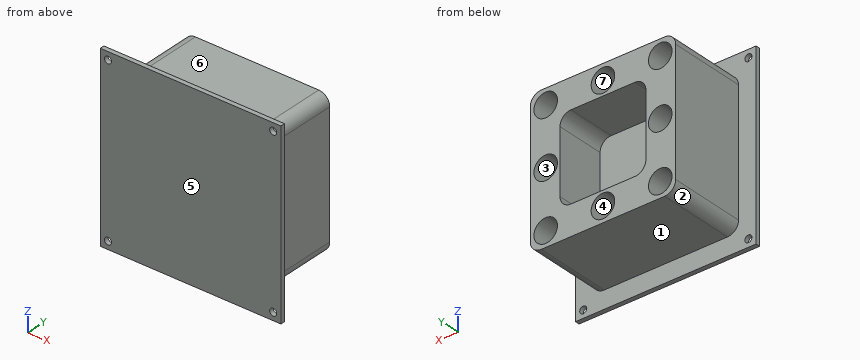
Autodesk Inventor part; units mm, degrees
ref_plane "YZ Plane" through (0, 0, 0) normal (1, 0, 0) x (0, 1, 0)
ref_plane "XZ Plane" through (0, 0, 0) normal (0, 1, 0) x (-1, 0, 0)
ref_plane "XY Plane" through (0, 0, 0) normal (0, 0, 1) x (1, 0, 0)
sketch "Sketch1" plane through (0, 0, 0) normal (0, 1, 0) x (-1, 0, 0)
  line L0 (28, 33) -> (-28, 33)
  line L1 (-33, 28) -> (-33, -28)
  line L2 (-28, -33) -> (28, -33)
  line L3 (33, -28) -> (33, 28)
  line L4 (33, 33) -> (-33, -33) construction
  line L5 (-33, 33) -> (33, -33) construction
  arc A0 (28, -33) -> (33, -28) centre (28, -28) ccw
  arc A1 (33, 28) -> (28, 33) centre (28, 28) ccw
  arc A2 (-28, 33) -> (-33, 28) centre (-28, 28) ccw
  arc A3 (-33, -28) -> (-28, -33) centre (-28, -28) ccw
  point P0 (0, 0)
  dimension "d0" = 66
  dimension "d1" = 66
  dimension "d4" = 5
extrude "Extrusion1" add sketch "Sketch1" along normal blind 35
sketch "Sketch2" plane through (0, 35, 0) normal (0, 1, 0) x (1, 0, 0)
  line L0 (0, 0) -> (-10, 0)
  line L1 (0, 0) -> (0, -10)
  circle A0 centre (26, 26) radius 5.35
  circle A1 centre (0, 26) radius 5.35
  circle A2 centre (-26, 26) radius 5.35
  circle A3 centre (26, 0) radius 5.35
  circle A4 centre (0, 0) radius 5.35
  circle A5 centre (-26, 0) radius 5.35
  circle A6 centre (26, -26) radius 5.35
  circle A7 centre (0, -26) radius 5.35
  circle A8 centre (-26, -26) radius 5.35
  dimension "d8" = 10
  dimension "d9" = 10
  dimension "d10" = 10.7
  dimension "d11" = 26
  dimension "d12" = 26
  dimension "d15" = 26
  dimension "d18" = 26
extrude "Extrusion2" cut sketch "Sketch2" against normal blind 35 contours A0 | A1 | A2 | A3 | A5 | A6 | A7 | A8
sketch "Sketch3" plane through (0, 35, 0) normal (0, 1, 0) x (1, 0, 0)
  line L0 (-14.5, -19.5) -> (14.5, -19.5)
  line L1 (19.5, -14.5) -> (19.5, 14.5)
  line L2 (14.5, 19.5) -> (-14.5, 19.5)
  line L3 (-19.5, 14.5) -> (-19.5, -14.5)
  line L4 (-19.5, -19.5) -> (19.5, 19.5) construction
  line L5 (19.5, -19.5) -> (-19.5, 19.5) construction
  arc A0 (-14.5, 19.5) -> (-19.5, 14.5) centre (-14.5, 14.5) ccw
  arc A1 (-19.5, -14.5) -> (-14.5, -19.5) centre (-14.5, -14.5) ccw
  arc A2 (14.5, -19.5) -> (19.5, -14.5) centre (14.5, -14.5) ccw
  arc A3 (19.5, 14.5) -> (14.5, 19.5) centre (14.5, 14.5) ccw
  point P0 (0, 0)
  dimension "d23" = 39
  dimension "d24" = 39
  dimension "d25" = 5
extrude "Extrusion3" cut sketch "Sketch3" against normal blind 22.3
sketch "Sketch4" plane through (0, 0, 0) normal (0, -1, 0) x (1, 0, 0)
  line L0 (37.5, 37.5) -> (-37.5, -37.5) construction
  line L1 (-37.5, 37.5) -> (37.5, -37.5) construction
  line L2 (-41, -38) -> (-41, 38)
  line L3 (41, -41) -> (-41, 41) construction
  line L4 (-41, -41) -> (41, 41) construction
  circle A0 centre (-37.5, 37.5) radius 1.6
  line L5 (38, 41) -> (-38, 41)
  line L6 (-38, -41) -> (38, -41)
  line L7 (41, -38) -> (41, 38)
  line L8 (41, 41) -> (-41, -41) construction
  line L9 (-41, 41) -> (41, -41) construction
  circle A1 centre (-37.5, -37.5) radius 1.6
  circle A2 centre (37.5, 37.5) radius 1.6
  circle A3 centre (37.5, -37.5) radius 1.6
  line L10 (-41, -38) -> (-41, -41)
  line L11 (-38, -41) -> (-41, -41)
  line L12 (-41, 38) -> (-41, 41)
  line L13 (-38, 41) -> (-41, 41)
  line L14 (38, 41) -> (41, 41)
  line L15 (41, 38) -> (41, 41)
  line L16 (41, -38) -> (41, -41)
  line L17 (41, -41) -> (38, -41)
  point P0 (0, 0)
  dimension "d28" = 75
  dimension "d29" = 75
  dimension "d31" = 82
  dimension "d56" = 3.2
  dimension "d68" = 75
  dimension "d71" = 75
extrude "Extrusion4" add sketch "Sketch4" along normal blind 2
properties part number "Aluminium Container" material "Aluminum 6061"
Input: part model. Units: mm. Frame: model coordinates. Face numbers are marked on the shaded views. A direction names the side the tool comes from. Give positions to 0.01 mm unless a question says otherwise; leave off trailing zeros. Loops run counter-clockwise (first coordinate to the right, second up) from the corner with the lowest first, then second, coordinate; pieces in that order, holes last. Notation, with made-up numbers: M 82,29.25 L 137,29.25 A13 ccw 137,37.25 Z; hole C 49,23.25 d5. An arc over 180 degrees is marked long. Use one line per item in the form item = value.
1. Pull-direction query (Z, two-part tool) for the marked faces 4, 5, 6 and 7; classes: released by +Z, released by -Z, zero draft, split by the parting line, or undercut.
Numbers:
face_4 = undercut
face_5 = zero draft
face_6 = released by +Z
face_7 = undercut
2. Section query B-B, the plane z = -37.5. Return the cut outline in (x, y).
Numbers:
outline = M -41,-2 L -39.1,-2 L -39.1,0 L -41,0 Z; M -35.9,-2 L 35.9,-2 L 35.9,0 L -35.9,0 Z; M 39.1,-2 L 41,-2 L 41,0 L 39.1,0 Z
3. Section query D-D, the plane z = 0. Return the cut outline in (x, y), and give its area (3 significant figures).
Numbers:
outline = M -41,-2 L 41,-2 L 41,0 L 33,0 L 33,35 L 31.35,35 L 31.35,0 L 20.65,0 L 20.65,35 L 19.5,35 L 19.5,12.7 L -19.5,12.7 L -19.5,35 L -20.65,35 L -20.65,0 L -31.35,0 L -31.35,35 L -33,35 L -33,0 L -41,0 Z
area = 855 mm²
4. Reachability of the marked faces 1, 2 and 3 from +Z, -Z, +X, -X, +Y, -Y: full face, straight path, thin tool, end or side. Return the list, or none.
Numbers:
face_1 = -Z, +X, -X, +Y
face_2 = -Z, -X, +Y
face_3 = +Y
5. First-contact query: pin 1 (2.5 mm diameter, centred on x = -37.5, z = -37.5, fed in from +Y); pin 2 (3 mm diameter, centred on x = 12, y = 4.5, fed in from -Z); pin 3 (4 mm diameter, centred on y = 10, z = -8, fed in from +X); pin 4 (5.5 mm diameter, centred on x = 1, z = 26, fed in from +Y). Flat tips, straight axial feed; report the tip coordinate or a pass-through.
Numbers:
pin_1 = through
pin_2 = -33
pin_3 = 33
pin_4 = 0
6. Section query C-C, the plane x = 26. Return the cut outline in (y, z).
Numbers:
outline = M -2,-41 L 0,-41 L 0,-33 L 35,-33 L 35,-31.35 L 0,-31.35 L 0,-20.65 L 35,-20.65 L 35,-5.35 L 0,-5.35 L 0,5.35 L 35,5.35 L 35,20.65 L 0,20.65 L 0,31.35 L 35,31.35 L 35,33 L 0,33 L 0,41 L -2,41 Z
7. Section query A-A, the plane y = 23. Count the separate pieces of the cut face and the enclosed holes in it, and give its area (3 significant figures).
Numbers:
separate_pieces = 1
enclosed_holes = 9
area = 2,120 mm²
8. Line query: L1, parallel to Z at x = -26, y = 22; L2, parallel to X at y = 32.5, z = -0.5. Output: solid intervals per line, ascending.
Numbers:
L1 = -33 to -31.35, -20.65 to -5.35, 5.35 to 20.65, 31.35 to 33
L2 = -33 to -31.33, -20.67 to -19.5, 19.5 to 20.67, 31.33 to 33
